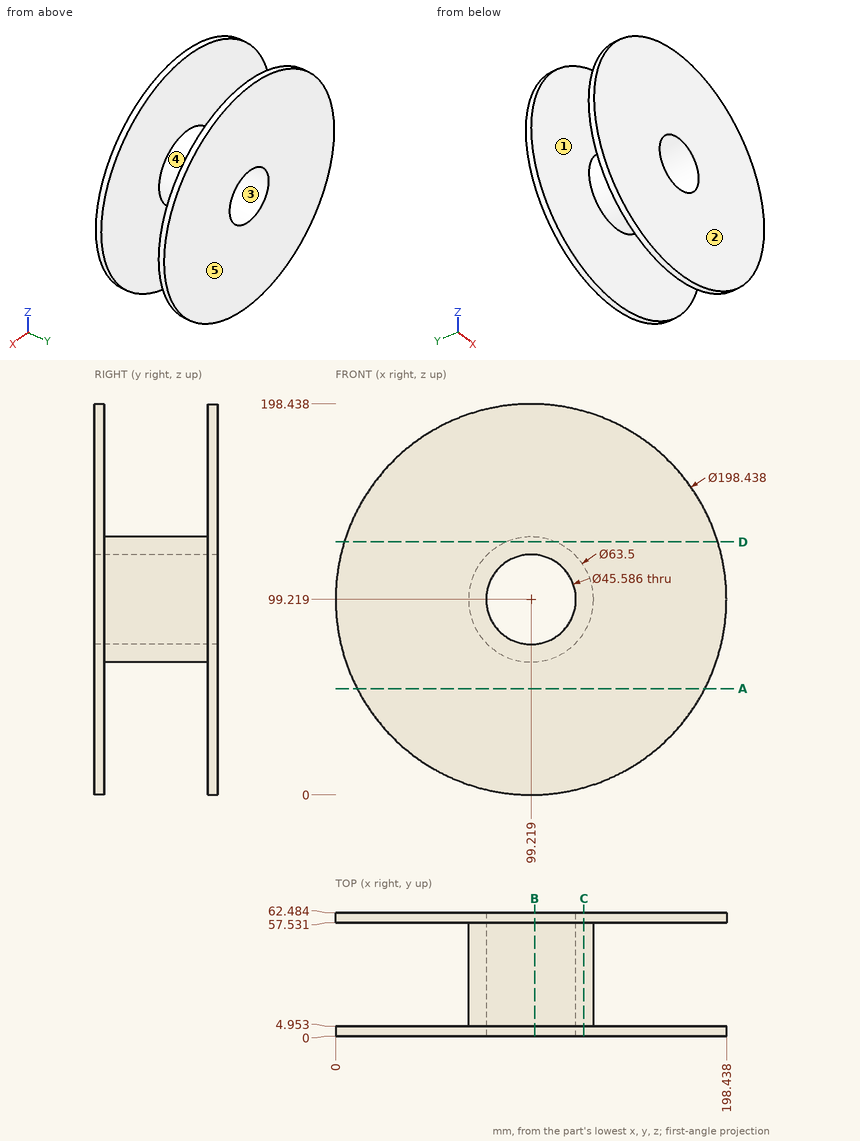
Answer from the drawing. Dimensions are ordinates in mm from the lowest x, y and z of the part. A direction names the side the tool comes from. Give positions to 0.01 mm unless a question says otherwise; leave off trailing zeros. Loops run counter-clockwise (first coordinate to the right, second up) from the corner with the lowest first, then second, coordinate; pieces in that order, holes last. Notation, with made-up numbers: (-30, -10) -> (-17, -10) arc R29 ccw to (-17, 27) -> close; hole circle Ø5 at (-6, -20.75). An arc over 180 degrees is marked (long way). Use a Markdown table: item, result.
Q1. Each of these flat-tipped pins is pushed along its axis until it touches: pin 1 (10 mm diameter, centred on y = 42.5, z = 91, fed in from +X) (1 decimal); pin 2 (4 mm diameter, centred on x = 118.5, y = 27.5, fed in from -Z) (1 decimal); pin 3 (5 mm diameter, centred on y = 53.5, z = 114, fed in from -X). Where does it stop, or does it pass through?
Solved:
| item | result |
|---|---|
| pin 1 | stops at x = 130.8 |
| pin 2 | stops at z = 72.6 |
| pin 3 | stops at x = 69.94 |
Q2. Section B-B, the plane x = 101 is taken. Determine the outline of the cut face in (y, z) (1 decimal), then the cut area to 3 significant figures.
Solved:
| item | result |
|---|---|
| outline | (0, 0) -> (5, 0) -> (5, 67.5) -> (57.5, 67.5) -> (57.5, 0) -> (62.5, 0) -> (62.5, 76.5) -> (0, 76.5) -> close; (0, 121.9) -> (62.5, 121.9) -> (62.5, 198.4) -> (57.5, 198.4) -> (57.5, 130.9) -> (5, 130.9) -> (5, 198.4) -> (0, 198.4) -> close |
| area | 2,460 mm^2 |
Q3. Section C-C, the plane x = 126 is taken. Determine the outline of the cut face in (y, z) (1 decimal).
Solved:
| item | result |
|---|---|
| outline | (0, 3.7) -> (5, 3.7) -> (5, 82.2) -> (57.5, 82.2) -> (57.5, 3.7) -> (62.5, 3.7) -> (62.5, 194.8) -> (57.5, 194.8) -> (57.5, 116.3) -> (5, 116.3) -> (5, 194.8) -> (0, 194.8) -> close |
Q4. A tool of negligible diameter and unlimited length cuts with its end or side. For the marked faces 1 and 2, from which of +Z, -Z, +X, -X, +Y, -Y can it reach the whole face along a straight path? Write none if from no direction.
Solved:
| item | result |
|---|---|
| face 1 | none |
| face 2 | +Z, -Z, +X, -X, -Y |
Q5. Section D-D, the plane z = 128.5 is taken. Determine the outline of the cut face in (x, y) (1 decimal).
Solved:
| item | result |
|---|---|
| outline | (4.4, 0) -> (194, 0) -> (194, 5) -> (111.5, 5) -> (111.5, 57.5) -> (194, 57.5) -> (194, 62.5) -> (4.4, 62.5) -> (4.4, 57.5) -> (86.9, 57.5) -> (86.9, 5) -> (4.4, 5) -> close |
Q6. Section A-A, the plane z = 54 is taken. Determine the outline of the cut face in (x, y) (1 decimal).
Solved:
| item | result |
|---|---|
| outline | (10.9, 0) -> (187.5, 0) -> (187.5, 5) -> (10.9, 5) -> close; (10.9, 57.5) -> (187.5, 57.5) -> (187.5, 62.5) -> (10.9, 62.5) -> close |
Q7. Determine the mould class of the marked faces 3, 4 and 5 for opening direction Y: pulls with the +Y half, pulls with the -Y half, needs draft (parallel to the pull), parting line crosses it, or undercut.
Solved:
| item | result |
|---|---|
| face 3 | needs draft |
| face 4 | undercut |
| face 5 | pulls with the +Y half |
Q8. Find the intervals of material crossed by line 1 along Y through (x, z) = (131, 174) (1 decimal); line 2 along Z through (x, y) = (98.5, 13); line 3 along Z through (x, y) = (97, 43) (1 decimal), in increasing order.
Solved:
| item | result |
|---|---|
| line 1 | y = 0 to 5, 57.5 to 62.5 |
| line 2 | z = 67.48 to 76.44, 122 to 130.96 |
| line 3 | z = 67.5 to 76.5, 121.9 to 130.9 |
